Autodesk Inventor part; units mm, degrees
ref_plane "YZ Plane" through (0, 0, 0) normal (1, 0, 0) x (0, 1, 0)
ref_plane "XZ Plane" through (0, 0, 0) normal (0, 1, 0) x (-1, 0, 0)
ref_plane "XY Plane" through (0, 0, 0) normal (0, 0, 1) x (1, 0, 0)
sketch "Sketch1" plane through (0, 0, 0) normal (0, 0, 1) x (1, 0, 0)
  line L0 (-7.8997, 15.5643) -> (8.1818, 15.5643)
  line L1 (8.1818, 15.5643) -> (8.1818, -14.4357)
  line L2 (8.1818, -14.4357) -> (-7.8997, -14.4357)
  line L3 (-7.8997, -14.4357) -> (-7.8997, 15.5643)
  line L4 (8.1818, 15.5643) -> (-7.8997, 15.5643)
  line L5 (-7.8997, 15.5643) -> (-7.8997, 23.2199)
  line L6 (-7.8997, 23.2199) -> (8.1818, 23.2199)
  line L7 (8.1818, 23.2199) -> (8.1818, 15.5643)
  point P0 (0, 0)
  dimension "d6" = 30
extrude "Extrusion1" add sketch "Sketch1" along normal blind 700 contours L0 L1 L2 L3
sketch "Sketch2" plane through (8.1818, -14.4357, 0) normal (1, 0, 0) x (0, 0, -1)
  line L0 (0, 0) -> (-700, 0)
  arc A0 (-30, 0) -> (-670, 0) centre (-350, -1691.6667) ccw
  line L1 (-30, 0) -> (-670, 0)
  line L2 (0, 30) -> (-700, 30)
  point P0 (0, 14.4357)
  dimension "d4" = 30
  dimension "d5" = 30
extrude "Extrusion2" cut sketch "Sketch2" against normal blind 90000
sketch "Sketch3" plane through (0, 0, 0) normal (0, 0, -1) x (-1, 0, 0)
  point P0 (0, 0)
extrude "Extrusion3" add sketch "Sketch1" along normal up to surface (700 mm away) contours L5 L6 L7 L0
equation "\"d5\" = d4"
properties part number "Group Bridge"
For this review, take the finished solid that the model builds, in its own axes (mm). Coordinates: 2 decimals unless noted, no trailing zeros. Write each loop counter-clockwise with the first axis right and the second up, starting at its lowest first coordinate (ties: lowest second). Pieces come first, ordered by that corner, then holes.
(1) Wall thickness on probe 1 along Y at (x, z) = (7.75, 354); probe 2 along Y at (x, z) = (3.25, 64): over which ranges is each line inside the solid? List them lowest first.
(2) The part is to be moulded in two halves that separate along Z. For faces 1 (the face through (0, 5, 0)), 2 (the face through (0, -14.436, 685)), 3 (the face through (0.25, 15.56, 345.49)), say which applies: +Z half, -Z half, draft (parallel to the pull), parting line (faces both ways), or undercut.
(3) Add section A-A on y = -5.5. Give the boundary of the cut face in (x, z), then the cut area to 3 significant figures.
(4) For pin 1 Ø8 at (y, z) = (9, 389.5) entering from +X, flat-tipped, find the tip position at first contact; note if it passes through.
(5) Add section C-C on z = 124. Give the boundary of the cut face in (x, y).
(6) Add section B-B on x = -3. Give the boundary of the cut face in (y, z), then the cut area to 3 significant figures.
(7) Add section D-D on z = 295. Give the boundary of the cut face in (x, y).
Answer sheet:
1. probe 1: y = 15.56 to 23.22
1. probe 2: y = -8.36 to 23.22
2. face 1: -Z half
2. face 2: draft
2. face 3: undercut
3. outline: (-7.9, 0) - (8.18, 0) - (8.18, 81.51) - (-7.9, 81.51) - close; (-7.9, 618.49) - (8.18, 618.49) - (8.18, 700) - (-7.9, 700) - close
3. area: 2,620 mm2
4. pin 1: passes through
5. outline: (-7.9, 0.67) - (8.18, 0.67) - (8.18, 23.22) - (-7.9, 23.22) - close
6. outline: (-14.44, 0) - (23.22, 0) - (23.22, 700) - (-14.44, 700) - (-14.44, 670) arc R1721.67 cw to (-14.44, 30) - close
6. area: 13,500 mm2
7. outline: (-7.9, 14.69) - (8.18, 14.69) - (8.18, 23.22) - (-7.9, 23.22) - close
